The model under review builds one solid part; all positions refer to its coordinate system, in mm. A direction names the side the tool comes from. Coordinates: 2 decimals unless noted, no trailing zeros. Order: outer loops, then holes, each group sorted by start corner. A loop starts at its lowest first (then second) coordinate and runs counter-clockwise, first axis right, second up. Notation, with made-up numbers: (48.5, 5.25) -> (106.5, 5.25) arc R20 cw to (106.5, 40.25) -> close; hole circle Ø4 at (17.5, -5.75). An arc over 180 degrees is marked (long way). Use one line per item in the form item = value.
from build123d import *

# Parameters (mm, degrees)
SKETCH_1_W             = 40
SKETCH_1_H             = 40
EXTRUDE_1_DEPTH        = 60
SKETCH_2_R             = 15.1
CUT_EXTRUDE_1_DEPTH    = 50
SKETCH_3_R             = 3
EXTRUDE_2_DEPTH        = 5
SKETCH_4_R             = 1.5
CUT_EXTRUDE_2_DEPTH    = 75.833147735
PATTERN_LINEAR_1_COUNT = 2
PATTERN_LINEAR_1_PITCH = 20


with BuildPart() as part:
    # 草圖1 → 填料-伸長1 (new body)
    with BuildSketch(Plane(origin=(0, 0, 0), x_dir=(1, 0, 0), z_dir=(0, 1, 0))):
        Rectangle(SKETCH_1_W, SKETCH_1_H)
    extrude(amount=EXTRUDE_1_DEPTH)

    # 草圖2 → 除料-伸長1 (cut)
    with BuildSketch(Plane(origin=(0, 60, 0), x_dir=(1, 0, 0), z_dir=(0, 1, 0))):
        with Locations(Location((0, 0, 0), (0, 0, 270))):
            Circle(SKETCH_2_R)
    extrude(amount=-CUT_EXTRUDE_1_DEPTH, mode=Mode.SUBTRACT)

    # 草圖3 → 填料-伸長2 (add)
    with BuildSketch(Plane.XY.offset(20)):
        with BuildLine():
            Line((-20, 0), (20, 0))
            ThreePointArc((20, 0), (0, -20), (-20, 0))
        make_face()
        with Locations((0, -8)):
            Circle(SKETCH_3_R, mode=Mode.SUBTRACT)
    extrude(amount=-EXTRUDE_2_DEPTH)

    # 草圖4 → 除料-伸長2 (cut, through all)
    with BuildSketch(Plane(origin=(20, 0, 0), x_dir=(0, 0, -1), z_dir=(1, 0, 0))):
        with Locations((0, 20)):
            Circle(SKETCH_4_R)
    cut_extrude_2 = extrude(amount=-CUT_EXTRUDE_2_DEPTH, mode=Mode.SUBTRACT)

    # 直線複製排列1: 除料-伸長2 ×2
    with Locations(*[(0, i * PATTERN_LINEAR_1_PITCH, 0) for i in range(1, PATTERN_LINEAR_1_COUNT)]):
        add(cut_extrude_2, mode=Mode.SUBTRACT)


solid = part.part
Item 1: Clearance check with flat-ended pins moving along their axes: pin 1 (2 mm diameter, centred on x = 9.5, z = -8, fed in from +Y); pin 2 (8 mm diameter, centred on x = 15.5, z = 3, fed in from -Y); pin 3 (6 mm diameter, centred on x = -9.5, y = -10, fed in from -Z). State where each tip first meets the part, or that it passes through.
Results found:
pin_1 = 10
pin_2 = 0
pin_3 = 15
Item 2: Tool access review of faces 5 (the face through (0, 0, -3)), 6 (the face through (-14.74, 35.35, -3.27)), 7 (the face through (-20, 30, 0)): name each direction out of +Z, -Z, +X, -X, +Y, -Y from which nothing blocks a thin tool from reaching the whole face with its end or side.
Results found:
face_5 = -Z, +X, -X, -Y
face_6 = +Y
face_7 = +Z, -Z, -X, +Y, -Y
Item 3: We need section B-B (z = 0). Write out the cut boundary in (x, y).
Results found:
outline = (-20, 0) -> (20, 0) -> (20, 18.5) -> (15.1, 18.5) -> (15.1, 10) -> (-15.1, 10) -> (-15.1, 18.5) -> (-20, 18.5) -> close; (-20, 21.5) -> (-15.1, 21.5) -> (-15.1, 38.5) -> (-20, 38.5) -> close; (-20, 41.5) -> (-15.1, 41.5) -> (-15.1, 60) -> (-20, 60) -> close; (15.1, 21.5) -> (20, 21.5) -> (20, 38.5) -> (15.1, 38.5) -> close; (15.1, 41.5) -> (20, 41.5) -> (20, 60) -> (15.1, 60) -> close
Item 4: We need section A-A (x = 0). Write out the cut boundary in (y, z).
Results found:
outline = (-20, 15) -> (-11, 15) -> (-11, 20) -> (-20, 20) -> close; (-5, 15) -> (0, 15) -> (0, -20) -> (60, -20) -> (60, -15.1) -> (10, -15.1) -> (10, 15.1) -> (60, 15.1) -> (60, 20) -> (-5, 20) -> close
Item 5: We need section C-C (y = 40). Write out the cut boundary in (x, z).
Results found:
outline = (-20, -20) -> (20, -20) -> (20, -1.5) -> (15.03, -1.5) arc R15.1 cw to (-15.03, -1.5) -> (-20, -1.5) -> close; (-20, 1.5) -> (-15.03, 1.5) arc R15.1 cw to (15.03, 1.5) -> (20, 1.5) -> (20, 20) -> (-20, 20) -> close
Item 6: We need section D-D (z = 16.5). Write out the cut boundary in (x, y).
Results found:
outline = (-20, 0) arc R20 ccw to (20, 0) -> (20, 60) -> (-20, 60) -> close; hole circle Ø6 at (0, -8)
Item 7: To check wall thickness, follow L1, parallel to Y at x = -16.85, z = 0; L2, parallel to Z at x = -18.05, y = 40; L3, parallel to X at y = 23.5, z = 0. State the ranges of each line that lie inside material, in increasing order. Write a range as from..to.
Results found:
L1 = 0..18.5, 21.5..38.5, 41.5..60
L2 = -20..-1.5, 1.5..20
L3 = -20..-15.1, 15.1..20
Item 8: Draft analysis for pull direction Z (two halves, no side actions). For faces 1 (the face through (0, 10, 0)), 2 (the face through (17.546, 21.487, 0.195)), 3 (the face through (20, 30, 0)), 4 (the face through (0, 21, 20)), state which applies: released by +Z, released by -Z, zero draft, split by the parting line, or undercut.
Results found:
face_1 = undercut
face_2 = undercut
face_3 = zero draft
face_4 = released by +Z
